Geometry: final body of the model. Coordinates: model frame, mm. Face numbers are marked on the shaded views. Round coordinates to 2 decimals unless told otherwise and drop trailing zeros. Loops run counter-clockwise (first coordinate to the right, second up) from the corner with the lowest first, then second, coordinate; pieces in that order, holes last. Notation, with made-up numbers: M 37.25,31 L 95.25,31 A18 cw 95.25,61 Z; hole C 69,89 d6. An arc over 180 degrees is marked long. Answer as a JSON object with one key per item and string values.
```python
from build123d import *

# Parameters (mm, degrees)
F0_R         = 17.8816960504
F0_R_2       = 10.3302818728
F1_DEPTH     = 25.4
F2_T1_DEPTH  = 162.5438125483
F2_T3_DEPTH  = 162.5438125483
F2_T6_ANGLE  = 188.1812058846
F2_T8_ANGLE  = 171.8187941154
F2_T10_ANGLE = 188.1812058846
F2_T12_ANGLE = 171.8187941154


# Not quite as in the source:
# - a fillet or chamfer that OpenCascade refuses, or shapes differently, is made with other operations: its cross-section is extruded or revolved along the edge and cut away or added


with BuildPart() as f1:
    # F0 (on Front) → F1 (new body)
    with BuildSketch(Plane.XZ):
        with BuildLine():
            ThreePointArc((-128.3244462029, -9.9682561267), (-108.7150059464, -0.8082782893), (-100.7286188282, 19.3077094309))
            ThreePointArc((-100.7286188282, 19.3077094309), (-108.4686726557, 39.1591179408), (-127.6033017493, 48.5321015922))
            ThreePointArc((-127.6033017493, 48.5321015922), (-159.38061509, 19.669202563), (-128.3244462029, -9.9682561267))
        make_face()
        with Locations((-130.0557309645, 19.3077094309)):
            Circle(F0_R, mode=Mode.SUBTRACT)
        with BuildLine():
            ThreePointArc((-127.6033017493, 48.5321015922), (-108.4686726557, 39.1591179408), (-100.7286188282, 19.3077094309))
            ThreePointArc((-100.7286188282, 19.3077094309), (-108.7150059464, -0.8082782893), (-128.3244462029, -9.9682561267))
            Line((-128.3244462029, -9.9682561267), (33.9358894089, -0.3727110744))
            ThreePointArc((33.9358894089, -0.3727110744), (15.1895627408, 17.5172445164), (34.3711913147, 34.9396553669))
            Line((34.3711913147, 34.9396553669), (-127.6033017493, 48.5321015922))
        make_face()
        with BuildLine():
            ThreePointArc((50.5934622257, 17.2990376807), (45.9213605892, 29.2818740087), (34.3711913147, 34.9396553669))
            ThreePointArc((34.3711913147, 34.9396553669), (15.1895627408, 17.5172445164), (33.9358894089, -0.3727110744))
            ThreePointArc((33.9358894089, -0.3727110744), (45.772667286, 5.1564943288), (50.5934622257, 17.2990376807))
        make_face()
        with Locations((32.89084004, 17.2990376807)):
            Circle(F0_R_2, mode=Mode.SUBTRACT)
    extrude(amount=F1_DEPTH)

    # F2: chamfer of 5.08 on 12 edges, made by hand

    # F2_s2 → F2_t1 (cut)
    with BuildSketch(Plane(origin=(31.219303845, 0, -2.6198366217), x_dir=(0, 1, 0), z_dir=(-0.9964974398, 0, 0.0836232768))):
        Polygon((-20.32, -37.691508766), (-25.4, -32.611508766), (-25.4, -37.691508766), align=None)
        Polygon((-5.08, -37.691508766), (0, -32.611508766), (0, -37.691508766), align=None)
    extrude(amount=F2_T1_DEPTH, mode=Mode.SUBTRACT)

    # F2_s4 → F2_t3 (cut)
    with BuildSketch(Plane(origin=(-128.4646756887, 0, -7.5969803622), x_dir=(0, 1, 0), z_dir=(0.9982559968, 0, 0.0590335916))):
        Polygon((-20.32, -2.3754185022), (-25.4, 2.7045814978), (-25.4, -2.3754185022), align=None)
        Polygon((-5.08, -2.3754185022), (0, 2.7045814978), (0, -2.3754185022), align=None)
    extrude(amount=F2_T3_DEPTH, mode=Mode.SUBTRACT)

    # F2_s5 → F2_t6 (revolve, cut)
    with BuildSketch(Plane(origin=(-130.755189219, 0, 10.9726096036), x_dir=(0, 1, 0), z_dir=(0.9964974398, 0, -0.0836232768))):
        Polygon((-20.32, 37.691508766), (-25.4, 32.611508766), (-25.4, 37.691508766), align=None)
    revolve(axis=Axis((-130.0557309645, -25.4, 19.3077094309), (0, -1, 0)), revolution_arc=F2_T6_ANGLE, mode=Mode.SUBTRACT)

    # F2_s7 → F2_t8 (revolve, cut)
    with BuildSketch(Plane(origin=(33.7956599231, 0, 1.9985646901), x_dir=(0, 1, 0), z_dir=(-0.9982559968, 0, -0.0590335916))):
        Polygon((-20.32, 2.3754185022), (-25.4, -2.7045814978), (-25.4, 2.3754185022), align=None)
    revolve(axis=Axis((32.89084004, -25.4, 17.2990376807), (0, -1, 0)), revolution_arc=F2_T8_ANGLE, mode=Mode.SUBTRACT)

    # F2_s9 → F2_t10 (revolve, cut)
    with BuildSketch(Plane(origin=(-130.755189219, 0, 10.9726096036), x_dir=(0, 1, 0), z_dir=(0.9964974398, 0, -0.0836232768))):
        Polygon((-5.08, 37.691508766), (0, 32.611508766), (0, 37.691508766), align=None)
    revolve(axis=Axis((-130.0557309645, 0, 19.3077094309), (0, -1, 0)), revolution_arc=F2_T10_ANGLE, mode=Mode.SUBTRACT)

    # F2_s11 → F2_t12 (revolve, cut)
    with BuildSketch(Plane(origin=(33.7956599231, 0, 1.9985646901), x_dir=(0, 1, 0), z_dir=(-0.9982559968, 0, -0.0590335916))):
        Polygon((-5.08, 2.3754185022), (0, -2.7045814978), (0, 2.3754185022), align=None)
    revolve(axis=Axis((32.89084004, 0, 17.2990376807), (0, -1, 0)), revolution_arc=F2_T12_ANGLE, mode=Mode.SUBTRACT)

    # F2_s13 → F2_t14 (revolve, cut)
    with BuildSketch(Plane.XY.offset(19.3077094309)):
        Polygon((-112.1740349142, -5.08), (-107.0940349142, 0), (-112.1740349142, 0), align=None)
    revolve(axis=Axis((-130.0557309645, 0, 19.3077094309), (0, -1, 0)), mode=Mode.SUBTRACT)

    # F2_s15 → F2_t16 (revolve, cut)
    with BuildSketch(Plane.XY.offset(19.3077094309)):
        Polygon((-112.1740349142, -20.32), (-107.0940349142, -25.4), (-112.1740349142, -25.4), align=None)
    revolve(axis=Axis((-130.0557309645, -25.4, 19.3077094309), (0, -1, 0)), mode=Mode.SUBTRACT)

    # F2_s17 → F2_t18 (revolve, cut)
    with BuildSketch(Plane.XY.offset(17.2990376807)):
        Polygon((43.2211219128, -20.32), (48.3011219128, -25.4), (43.2211219128, -25.4), align=None)
    revolve(axis=Axis((32.89084004, -25.4, 17.2990376807), (0, -1, 0)), mode=Mode.SUBTRACT)

    # F2_s19 → F2_t20 (revolve, cut)
    with BuildSketch(Plane.XY.offset(17.2990376807)):
        Polygon((43.2211219128, -5.08), (48.3011219128, 0), (43.2211219128, 0), align=None)
    revolve(axis=Axis((32.89084004, 0, 17.2990376807), (0, -1, 0)), mode=Mode.SUBTRACT)


solid = f1.part
```
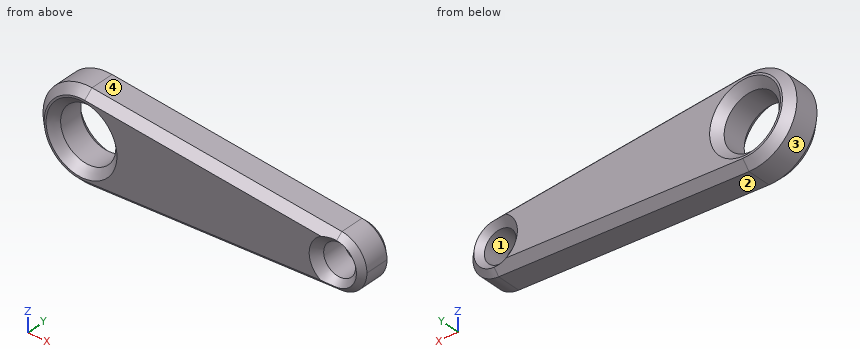
1) Cut plane A-A on x = -10.5. Return the cut outline in (y, z), and give its area (3 significant figures).
Geometry results:
{"outline": "M -25.4,2.09 L -20.32,-3 L -5.08,-3 L 0,2.09 L 0,33.61 L -5.08,38.71 L -20.32,38.71 L -25.4,33.61 Z", "area": "1,010 mm2"}
2) First-contact query: pin 1 (1.5 mm diameter, centred on x = -39, y = -8.5, fed in from +Z); pin 2 (1.5 mm diameter, centred on y = -18, z = 22, fed in from -X); pin 3 (10 mm diameter, centred on x = -28.5, y = -6, fed in from -Z); pin 4 (12.5 mm diameter, centred on x = 32.89, z = 17.3, fed in from +Y). Flat tips, straight axial feed; report the tip coordinate or a pass-through.
Geometry results:
{"pin 1": "z = 41.16", "pin 2": "x = -159.32", "pin 3": "z = -4.36", "pin 4": "through"}
3) Cut plane B-B on z = 14.5. Count the separate pieces of the cut face and the enclosed holes in it, and give its area (3 significant figures).
Geometry results:
{"separate pieces": "3", "enclosed holes": "0", "area": "3,780 mm2"}
4) Cut plane D-D on x = -88. Return the cut outline in (y, z).
Geometry results:
{"outline": "M -25.4,-2.49 L -20.32,-7.58 L -5.08,-7.58 L 0,-2.49 L 0,40.11 L -5.08,45.21 L -20.32,45.21 L -25.4,40.11 Z"}
5) Line query: probe 1 along X at (y, z) = (-8.5, 14); probe 2 along X at (y, z) = (-5.25, 10.5); probe 3 along X at (y, z) = (-15.75, 28.5) (3 decimals). Output: solid intervals per line, ascending.
Geometry results:
{"probe 1": "-158.9 to -147.13, -112.98 to 23.1, 42.68 to 50.28", "probe 2": "-158.03 to -145.62, -114.49 to 25.11, 40.67 to 49.24", "probe 3": "-157.905 to -145.394, -114.718 to 46.599"}
6) Pull-direction query (Z, two-part tool) for the marked faces 1, 2, 3 and 4; classes: +Z half, -Z half, draft (parallel to the pull), parting line (faces both ways), or undercut.
Geometry results:
{"face 1": "undercut", "face 2": "-Z half", "face 3": "parting line", "face 4": "+Z half"}
7) Cut plane C-C on y = -14.5. Return the cut outline in (x, z).
Geometry results:
{"outline": "M -128.32,-9.97 L 33.94,-0.37 A17.7 ccw 34.37,34.94 L -127.6,48.53 A29.33 ccw long Z; hole C -130.06,19.31 d35.76; hole C 32.89,17.3 d20.66"}
